from build123d import *

# Parameters (mm, degrees)
SKETCH1_R           = 5
BOSS_EXTRUDE1_DEPTH = 19
SKETCH2_R           = 4
BOSS_EXTRUDE2_DEPTH = 15
BOSS_EXTRUDE3_START = -53
SKETCH2_2_R         = 4
BOSS_EXTRUDE3_DEPTH = 15
CHAMFER2_SIZE       = 0.5
SKETCH3_R           = 3.1
BOSS_EXTRUDE4_DEPTH = 12
CHAMFER3_SIZE       = 0.5


# Read off the part's stored shape, not the designer's step: M6 Machine Threads Stud1, M6 Machine Threads Stud2
with BuildPart() as part:
    # Sketch1 → Boss-Extrude1 (new, symmetric)
    with BuildSketch(Plane(origin=(0, 0, 0), x_dir=(1, 0, 0), z_dir=(0, 1, 0))):
        with Locations(Location((0, 0, 0), (0, 0, 270))):
            Circle(SKETCH1_R)
    extrude(amount=BOSS_EXTRUDE1_DEPTH, both=True)

    # Sketch2 → Boss-Extrude2 (add)
    with BuildSketch(Plane(origin=(0, 19, 0), x_dir=(1, 0, 0), z_dir=(0, 1, 0))):
        with Locations(Location((0, 0, 0), (0, 0, 270))):
            Circle(SKETCH2_R)
    extrude(amount=BOSS_EXTRUDE2_DEPTH)

    # Sketch2<2> → Boss-Extrude3 (add)
    with BuildSketch(Plane(origin=(0, 19, 0), x_dir=(1, 0, 0), z_dir=(0, 1, 0)).offset(BOSS_EXTRUDE3_START)):
        with Locations(Location((0, 0, 0), (0, 0, 270))):
            Circle(SKETCH2_2_R)
    extrude(amount=BOSS_EXTRUDE3_DEPTH)

    # Chamfer2
    chamfer2_edges = [part.edges().sort_by_distance(p)[0] for p in [
        (0, -19, -5),
        (0, 19, -5),
    ]]
    chamfer(chamfer2_edges, length=CHAMFER2_SIZE)

    # Sketch3 → Boss-Extrude4 (add)
    with BuildSketch(Plane(origin=(0, 34, 0), x_dir=(1, 0, 0), z_dir=(0, 1, 0))):
        with Locations(Location((0, 0, 0), (0, 0, 270))):
            Circle(SKETCH3_R)
    boss_extrude4 = extrude(amount=BOSS_EXTRUDE4_DEPTH)

    # M6 Machine Threads Stud1 outline → M6 Machine Threads Stud1 (revolve, cut)
    with BuildSketch(Plane.XY):
        with BuildLine():
            Line((3.1, 46), (2.4455, 46))
            Line((2.4455, 46), (3, 45.4455))
            Line((3, 45.4455), (3, 36.939230485))
            Line((3, 36.939230485), (2.053589838, 35.3))
            ThreePointArc((2.053589838, 35.3), (2.013629669, 35.203527618), (2, 35.1))
            Line((2, 35.1), (2, 34.4))
            ThreePointArc((2, 34.4), (2.117157288, 34.117157288), (2.4, 34))
            Line((2.4, 34), (3.1, 34))
            Line((3.1, 34), (3.1, 46))
        make_face()
    revolve(axis=Axis((0, 0, 0), (0, 1, 0)), mode=Mode.SUBTRACT)

    # Mirror1: Boss-Extrude4 across plane
    add(boss_extrude4.mirror(Plane.ZX))

    # M6 Machine Threads Stud2 outline → M6 Machine Threads Stud2 (revolve, cut)
    with BuildSketch(Plane.XY):
        with BuildLine():
            Line((2.4455, -46), (3.1, -46))
            Line((3.1, -46), (3.1, -34))
            Line((3.1, -34), (2.4, -34))
            ThreePointArc((2.4, -34), (2.117157288, -34.117157288), (2, -34.4))
            Line((2, -34.4), (2, -35.1))
            ThreePointArc((2, -35.1), (2.013629669, -35.203527618), (2.053589838, -35.3))
            Line((2.053589838, -35.3), (3, -36.939230485))
            Line((3, -36.939230485), (3, -45.4455))
            Line((3, -45.4455), (2.4455, -46))
        make_face()
    revolve(axis=Axis((0, 0, 0), (0, 1, 0)), mode=Mode.SUBTRACT)

    # Chamfer3
    chamfer3_edges = [part.edges().sort_by_distance(p)[0] for p in [
        (0, -34, -4),
        (0, 34, -4),
    ]]
    chamfer(chamfer3_edges, length=CHAMFER3_SIZE)


solid = part.part
The listing builds one solid part. Answer for the finished solid, in the listing's coordinates (mm). A direction names the side the tool comes from. Round coordinates to 2 decimals unless told otherwise and drop trailing zeros. Write each loop counter-clockwise with the first axis right and the second up, starting at its lowest first coordinate (ties: lowest second). Pieces come first, ordered by that corner, then holes. Notation, with made-up numbers: (33.5, 68.5) - (44.5, 68.5) arc R19 cw to (44.5, 96.5) - close; hole circle Ø8 at (63, 24.25). An arc over 180 degrees is marked (long way). Use a Markdown table: item, result. Add a question column.
1. The part is cut by section B-B (y = 17). Write down the section's boundary in (x, z), and give its area (3 significant figures).
2. The part is cut by section A-A (y = -24). Write down the section's boundary in (x, z), and give its area (3 significant figures).
3. For a pull along Y with two mould halves and no side action, classify faces 5 (the face through (0, -46, 0)), 6 (the face through (-3, 19, -3)), 7 (the face through (-0.434, 34.745, 1.952)) as +Y half, -Y half, draft (parallel to the pull), parting line (faces both ways), or undercut.
4. Flat-ended cylindrical pins translate along their axes: P1, Ø1.5, axis at x = -1, z = 3.5, coming from the -Y side; P2, Ø2, axis at x = 1.5, y = -36.5, coming from the -Z side; P3, Ø1.5, axis at x = -0.5, z = 4, coming from the +Y side. Find the tip coordinate at first contact, or state that the pin passes through.
5. Consider line 1 (Y direction, x = -1.5, z = 2.25); line 2 (Y direction, x = -2.5, z = 1.25); line 3 (Y direction, x = -2.5, z = 2.25). Determine where each line is inside the solid, lowest interval first.
6. A tool of negligible diameter and unlimited length cuts with its end or side. For faces 1 (the face through (-0.434, -34.755, 1.952)), 2 (the face through (-3.905, 26.148, -0.867)), 3 (the face through (-3, -41, 0)), 4 (the face through (-4.88, 0.26, -1.08)), from which of +Z, -Z, +X, -X, +Y, -Y can it reach the whole face along a straight path? Write none if from no direction.
Reported:
| question | item | result |
|---|---|---|
| 1 | outline | circle Ø10 at (0, 0) |
| 1 | area | 78.5 mm^2 |
| 2 | outline | circle Ø8 at (0, 0) |
| 2 | area | 50.3 mm^2 |
| 3 | face 5 | -Y half |
| 3 | face 6 | +Y half |
| 3 | face 7 | undercut |
| 4 | P1 | y = -45.56 |
| 4 | P2 | z = -2.94 |
| 4 | P3 | y = 34 |
| 5 | line 1 | -45.74 to -36.43, -34 to 34, 36.43 to 45.74 |
| 5 | line 2 | -45.65 to -36.58, -34 to 34, 36.58 to 45.65 |
| 5 | line 3 | -34 to 34 |
| 6 | face 1 | none |
| 6 | face 2 | +Y |
| 6 | face 3 | -Y |
| 6 | face 4 | +Y, -Y |
